from build123d import *

# Parameters (mm, degrees)
SKETCH1_W                 = 629.92
SKETCH1_H                 = 101.6
BASE_FLANGE1_DEPTH        = 3.175
EDGE_FLANGE1_DEPTH        = 617.22
EDGE_FLANGE2_DEPTH        = 101.6
EDGE_FLANGE2_BEND_DEPTH   = 101.6
EDGE_FLANGE3_DEPTH        = 630.46
EDGE_FLANGE4_DEPTH        = 630.46
EDGE_FLANGE5_DEPTH        = 630.46
EDGE_FLANGE6_DEPTH        = 58.706
EDGE_FLANGE6_BEND_DEPTH   = 58.706
EDGE_FLANGE6_BEND_2_DEPTH = 398.304
EDGE_FLANGE6_BEND_3_DEPTH = 398.304


# Sheet-metal steps are written as plain solids
with BuildPart() as part:
    # Sketch1 → Base-Flange1 (new body)
    with BuildSketch(Plane.XY):
        Rectangle(SKETCH1_W, SKETCH1_H)
    extrude(amount=-BASE_FLANGE1_DEPTH)

    # Edge-Flange1 section (across the edge) → Edge-Flange1 (add)
    with BuildSketch(Plane(origin=(-308.61, 52.07, -3.175), x_dir=(0, -1, 0), z_dir=(1, 0, 0))):
        with BuildLine():
            Line((-3.175, 1), (-3.175, 17.78))
            Line((-3.175, 17.78), (0, 17.78))
            Line((0, 17.78), (0, 1))
            ThreePointArc((0, 1), (0.292893219, 0.292893219), (1, 0))
            Line((1, 0), (1.27, 0))
            Line((1.27, 0), (1.27, -3.175))
            Line((1.27, -3.175), (1, -3.175))
            ThreePointArc((1, -3.175), (-1.952170811, -1.952170811), (-3.175, 1))
        make_face()
    extrude(amount=EDGE_FLANGE1_DEPTH)

    # Edge-Flange2 section (across the edge) → Edge-Flange2 (add)
    with BuildSketch(Plane(origin=(-316.23, -50.8, -3.175), x_dir=(1, 0, 0), z_dir=(0, 1, 0))):
        with BuildLine():
            Line((-3.175, 1), (-3.175, 17.78))
            Line((-3.175, 17.78), (0, 17.78))
            Line((0, 17.78), (0, 1))
            ThreePointArc((0, 1), (0.292893219, 0.292893219), (1, 0))
            Line((1, 0), (1.27, 0))
            Line((1.27, 0), (1.27, -3.175))
            Line((1.27, -3.175), (1, -3.175))
            ThreePointArc((1, -3.175), (-1.952170811, -1.952170811), (-3.175, 1))
        make_face()
    extrude(amount=EDGE_FLANGE2_DEPTH)

    # Edge-Flange2 section 2 (across the edge) → Edge-Flange2 bend (add)
    with BuildSketch(Plane(origin=(316.23, 50.8, -3.175), x_dir=(-1, 0, 0), z_dir=(0, -1, 0))):
        with BuildLine():
            Line((-3.175, 1), (-3.175, 17.78))
            Line((-3.175, 17.78), (0, 17.78))
            Line((0, 17.78), (0, 1))
            ThreePointArc((0, 1), (0.292893219, 0.292893219), (1, 0))
            Line((1, 0), (1.27, 0))
            Line((1.27, 0), (1.27, -3.175))
            Line((1.27, -3.175), (1, -3.175))
            ThreePointArc((1, -3.175), (-1.952170811, -1.952170811), (-3.175, 1))
        make_face()
    extrude(amount=EDGE_FLANGE2_BEND_DEPTH)

    # Edge-Flange3 section (across the edge) → Edge-Flange3 (add)
    with BuildSketch(Plane(origin=(315.23, -52.07, -3.175), x_dir=(0, 1, 0), z_dir=(-1, 0, 0))):
        with BuildLine():
            Line((-3.175, 1), (-3.175, 77.216))
            Line((-3.175, 77.216), (0, 77.216))
            Line((0, 77.216), (0, 1))
            ThreePointArc((0, 1), (0.292893219, 0.292893219), (1, 0))
            Line((1, 0), (1.27, 0))
            Line((1.27, 0), (1.27, -3.175))
            Line((1.27, -3.175), (1, -3.175))
            ThreePointArc((1, -3.175), (-1.952170811, -1.952170811), (-3.175, 1))
        make_face()
    extrude(amount=EDGE_FLANGE3_DEPTH)

    # Edge-Flange4 section (across the edge) → Edge-Flange4 (add)
    with BuildSketch(Plane(origin=(-315.23, -55.245, -81.661), x_dir=(0, 0, 1), z_dir=(1, 0, 0))):
        with BuildLine():
            Line((-3.175, 1), (-3.175, 399.034))
            Line((-3.175, 399.034), (0, 399.034))
            Line((0, 399.034), (0, 1))
            ThreePointArc((0, 1), (0.292893219, 0.292893219), (1, 0))
            Line((1, 0), (1.27, 0))
            Line((1.27, 0), (1.27, -3.175))
            Line((1.27, -3.175), (1, -3.175))
            ThreePointArc((1, -3.175), (-1.952170811, -1.952170811), (-3.175, 1))
        make_face()
    extrude(amount=EDGE_FLANGE4_DEPTH)

    # Edge-Flange5 section (across the edge) → Edge-Flange5 (add)
    with BuildSketch(Plane(origin=(315.23, -455.549, -84.836), x_dir=(0, 1, 0), z_dir=(-1, 0, 0))):
        with BuildLine():
            Line((-3.175, 1), (-3.175, 17.78))
            Line((-3.175, 17.78), (0, 17.78))
            Line((0, 17.78), (0, 1))
            ThreePointArc((0, 1), (0.292893219, 0.292893219), (1, 0))
            Line((1, 0), (1.27, 0))
            Line((1.27, 0), (1.27, -3.175))
            Line((1.27, -3.175), (1, -3.175))
            ThreePointArc((1, -3.175), (-1.952170811, -1.952170811), (-3.175, 1))
        make_face()
    extrude(amount=EDGE_FLANGE5_DEPTH)

    # Edge-Flange6 section (across the edge) → Edge-Flange6 (add)
    with BuildSketch(Plane(origin=(-316.5, -52.07, -80.661), x_dir=(1, 0, 0), z_dir=(0, 0, 1))):
        with BuildLine():
            Line((-3.175, 1), (-3.175, 17.78))
            Line((-3.175, 17.78), (0, 17.78))
            Line((0, 17.78), (0, 1))
            ThreePointArc((0, 1), (0.292893219, 0.292893219), (1, 0))
            Line((1, 0), (1.27, 0))
            Line((1.27, 0), (1.27, -3.175))
            Line((1.27, -3.175), (1, -3.175))
            ThreePointArc((1, -3.175), (-1.952170811, -1.952170811), (-3.175, 1))
        make_face()
    extrude(amount=EDGE_FLANGE6_DEPTH)

    # Edge-Flange6 section 2 (across the edge) → Edge-Flange6 bend (add)
    with BuildSketch(Plane(origin=(316.5, -52.07, -21.955), x_dir=(-1, 0, 0), z_dir=(0, 0, -1))):
        with BuildLine():
            Line((-3.175, 1), (-3.175, 17.78))
            Line((-3.175, 17.78), (0, 17.78))
            Line((0, 17.78), (0, 1))
            ThreePointArc((0, 1), (0.292893219, 0.292893219), (1, 0))
            Line((1, 0), (1.27, 0))
            Line((1.27, 0), (1.27, -3.175))
            Line((1.27, -3.175), (1, -3.175))
            ThreePointArc((1, -3.175), (-1.952170811, -1.952170811), (-3.175, 1))
        make_face()
    extrude(amount=EDGE_FLANGE6_BEND_DEPTH)

    # Edge-Flange6 section 3 (across the edge) → Edge-Flange6 bend 2 (add)
    with BuildSketch(Plane(origin=(-316.5, -454.549, -84.836), x_dir=(1, 0, 0), z_dir=(0, 1, 0))):
        with BuildLine():
            Line((-3.175, 1), (-3.175, 17.78))
            Line((-3.175, 17.78), (0, 17.78))
            Line((0, 17.78), (0, 1))
            ThreePointArc((0, 1), (0.292893219, 0.292893219), (1, 0))
            Line((1, 0), (1.27, 0))
            Line((1.27, 0), (1.27, -3.175))
            Line((1.27, -3.175), (1, -3.175))
            ThreePointArc((1, -3.175), (-1.952170811, -1.952170811), (-3.175, 1))
        make_face()
    extrude(amount=EDGE_FLANGE6_BEND_2_DEPTH)

    # Edge-Flange6 section 4 (across the edge) → Edge-Flange6 bend 3 (add)
    with BuildSketch(Plane(origin=(316.5, -56.245, -84.836), x_dir=(-1, 0, 0), z_dir=(0, -1, 0))):
        with BuildLine():
            Line((-3.175, 1), (-3.175, 17.78))
            Line((-3.175, 17.78), (0, 17.78))
            Line((0, 17.78), (0, 1))
            ThreePointArc((0, 1), (0.292893219, 0.292893219), (1, 0))
            Line((1, 0), (1.27, 0))
            Line((1.27, 0), (1.27, -3.175))
            Line((1.27, -3.175), (1, -3.175))
            ThreePointArc((1, -3.175), (-1.952170811, -1.952170811), (-3.175, 1))
        make_face()
    extrude(amount=EDGE_FLANGE6_BEND_3_DEPTH)


solid = part.part
Work out the finished part from the listing and answer in its coordinate system (mm). A direction names the side the tool comes from. Coordinates: 2 decimals unless noted, no trailing zeros. Write each loop counter-clockwise with the first axis right and the second up, starting at its lowest first coordinate (ties: lowest second). Pieces come first, ordered by that corner, then holes. Notation, with made-up numbers: M 15,-11.75 L 47,-11.75 A15 ccw 47,-0.75 Z; hole C 24,37.25 d7. An arc over 180 degrees is marked long. Write item = value, one per line.
1. Straight lines are drawn through the part: line 1 (X direction, y = -41, z = -55) (3 decimals); line 2 (Y direction, x = 228, z = -6) (3 decimals); line 3 (Y direction, x = 268, z = -35) (3 decimals). For each, find the intervals that lie inside material, in ascending order. Write a range as from..to.
Solution:
line_1 = -319.675..-316.5, 316.5..319.675
line_2 = -55.245..-52.07, 52.07..55.245
line_3 = -55.245..-52.07
2. The part is cut by section B-B (x = -134). Determine the outline of the cut face in (y, z) (3 decimals), then the cut area to 3 significant figures.
Solution:
outline = M -458.724,-102.616 L -455.549,-102.616 L -455.549,-85.836 A1 cw -454.549,-84.836 L -56.245,-84.836 A4.175 ccw -52.07,-80.661 L -52.07,-4.175 A1 cw -51.07,-3.175 L 51.07,-3.175 A1 cw 52.07,-4.175 L 52.07,-20.955 L 55.245,-20.955 L 55.245,-4.175 A4.175 ccw 51.07,0 L -51.07,0 A4.175 ccw -55.245,-4.175 L -55.245,-80.661 A1 cw -56.245,-81.661 L -454.549,-81.661 A4.175 ccw -458.724,-85.836 Z
area = 1,990 mm2
3. The part is cut by section C-C (z = -36.5). Determine the outline of the cut face in (x, y) (3 decimals).
Solution:
outline = M -319.675,-51.07 A4.175 ccw -315.5,-55.245 L 315.5,-55.245 A4.175 ccw 319.675,-51.07 L 319.675,-34.29 L 316.5,-34.29 L 316.5,-51.07 A1 cw 315.5,-52.07 L -315.5,-52.07 A1 cw -316.5,-51.07 L -316.5,-34.29 L -319.675,-34.29 Z
4. Flat-ended cylindrical pins translate along their axes: pin 1 (8 mm diameter, centred on x = -32.5, z = -91.5, fed in from +Y); pin 2 (5 mm diameter, centred on x = -72.5, y = -28.5, fed in from -Z) (3 decimals); pin 3 (3 mm diameter, centred on x = 207.5, z = -28, fed in from -Y) (3 decimals). Find the tip coordinate at first contact, or state that the pin passes through.
Solution:
pin_1 = -455.55
pin_2 = -3.175
pin_3 = -55.245
5. For faces 4 (the face through (4, -253, -84.836)), 5 (the face through (4, -52.07, -42)), 6 (the face through (-316.23, -1, -13)), determine the directions among +Z, -Z, +X, -X, +Y, -Y from which every point of the face is accessible in a straight line to the end or side of a thin tool.
Solution:
face_4 = -Z, +Y
face_5 = -Z
face_6 = -Z, +Y, -Y
6. Determine the mould class of faces 1 (the face through (4, -458.724, -94)), 2 (the face through (-319.405, -1, -12)), 3 (the face through (-4, 52.07, -13)) for opening direction Y: released by +Y, released by -Y, zero draft, split by the parting line, or undercut.
Solution:
face_1 = released by -Y
face_2 = zero draft
face_3 = undercut
7. The part is cut by section A-A (y = 17). Determine the outline of the cut face in (x, z) (3 decimals).
Solution:
outline = M -319.405,-20.955 L -316.23,-20.955 L -316.23,-4.175 A1 cw -315.23,-3.175 L 315.23,-3.175 A1 cw 316.23,-4.175 L 316.23,-20.955 L 319.405,-20.955 L 319.405,-4.175 A4.175 ccw 315.23,0 L -315.23,0 A4.175 ccw -319.405,-4.175 Z
